Geometry: final body of the model. Coordinates: model frame, mm. Round coordinates to 2 decimals unless told otherwise and drop trailing zeros. Write each loop counter-clockwise with the first axis right and the second up, starting at its lowest first coordinate (ties: lowest second). Pieces come first, ordered by that corner, then holes. Notation, with made-up numbers: (-25.5, 72) - (26.5, 72) arc R20 ccw to (26.5, 93) - close; hole circle Ø2 at (42, 52.25). An arc over 180 degrees is marked (long way). Write each question's results on one line, items separated by ' | '.
from build123d import *

# Parameters (mm, degrees)
SKETCH_1_W          = 44.8
SKETCH_1_H          = 2000
EXTRUDE_1_DEPTH     = 10
CUT_EXTRUDE_2_DEPTH = 3329.04869605
EXTRUDE_2_DEPTH     = 44.8
CUT_EXTRUDE_3_DEPTH = 8.96


with BuildPart() as part:
    # 草图1 → 凸台-拉伸1 (new body)
    with BuildSketch(Plane(origin=(915.505475204, 0, 2515.33062051), x_dir=(-0.9396926207859093, 0, 0.3420201433256663), z_dir=(-0.3420201433256663, 0, -0.9396926207859093))):
        with Locations((-82.338659964, -943.731460395)):
            Rectangle(SKETCH_1_W, SKETCH_1_H)
    extrude(amount=-EXTRUDE_1_DEPTH)

    # 草图2 → 切除-拉伸2 (cut, through all)
    with BuildSketch(Plane(origin=(56.323916468, 0, -20.500229072), x_dir=(0.34202014332566644, 0, 0.9396926207859093), z_dir=(-0.9396926207859092, 0, 0.3420201433256664))):
        with BuildLine():
            Line((2678.733687242, 56.268539605), (2678.733687242, 49.653408924))
            Line((2678.733687242, 49.653408924), (2684.784186307, 49.653408924))
            ThreePointArc((2684.784186307, 49.653408924), (2684.783800485, 49.701723134), (2684.78264312, 49.750025021))
            Line((2684.78264312, 49.750025021), (2684.784186307, 56.268539605))
            Line((2684.784186307, 56.268539605), (2678.733687242, 56.268539605))
        make_face()
        with BuildLine():
            Line((2684.784186307, 49.653408924), (2678.733687242, 49.653408924))
            ThreePointArc((2678.733687242, 49.653408924), (2681.758936775, 46.628159392), (2684.784186307, 49.653408924))
        make_face()
    extrude(amount=-CUT_EXTRUDE_2_DEPTH, mode=Mode.SUBTRACT)

    # 草图3 → 凸台-拉伸2 (add)
    with BuildSketch(Plane(origin=(56.323916468, 0, -20.500229072), x_dir=(0.34202014332566644, 0, 0.9396926207859093), z_dir=(-0.9396926207859092, 0, 0.3420201433256664))):
        with BuildLine():
            Line((2678.733687242, 49.653408924), (2678.733687242, 56.268539605))
            Line((2678.733687242, 56.268539605), (2684.784186307, 56.268539605))
            Line((2684.784186307, 56.268539605), (2684.784186307, 49.653408924))
            ThreePointArc((2684.784186307, 49.653408924), (2681.758936775, 46.628159392), (2678.733687242, 49.653408924))
        make_face()
    extrude(amount=-EXTRUDE_2_DEPTH)

    # 草图4 → 切除-拉伸3 (cut)
    with BuildSketch(Plane(origin=(0, 56.268539605, 0), x_dir=(1, 0, 0), z_dir=(0, 1, 0))):
        Polygon((995.8288615, -2496.737076507), (996.29870781, -2496.566066436), (992.878506377, -2487.169140228), (992.408660067, -2487.340150299), align=None)
        Polygon((992.878506377, -2487.169140228), (996.29870781, -2496.566066436), (996.768554121, -2496.395056364), (993.348352687, -2486.998130156), align=None)
    extrude(amount=-CUT_EXTRUDE_3_DEPTH, mode=Mode.SUBTRACT)


solid = part.part
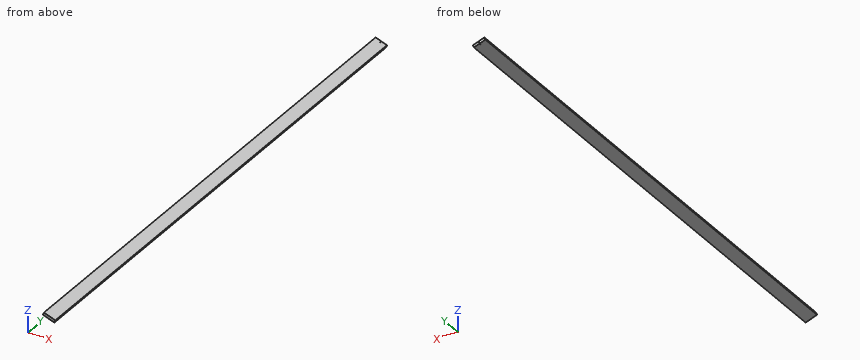
Q1. Section query A-A, the plane y = -304.5. Return loops of the section in (x, z), plus the area to 3 significant figures.
Answer block:
outline: (971.83, 2494.83) - (1013.93, 2479.51) - (1017.35, 2488.9) - (975.25, 2504.23) - close | area: 448 mm2
Q2. Pin query (flat end, axial travel): pin 1 (2 mm diameter, centred on x = 994.5, y = -587, fed in from -Z) (3 decimals); pin 2 (1.5 mm diameter, centred on x = 990, y = -1442.5, fed in from +Z); pin 3 (1.5 mm diameter, centred on x = 1004, y = -907.5, fed in from -Z). Return the tip coordinate at first contact, or that it passes through.
Answer block:
pin 1: z = 2486.215 | pin 2: z = 2499.13 | pin 3: z = 2482.85
Q3. Ray query, line 1 along Z through (x, y) = (990.5, -707.5); line 2 along Z through (x, y) = (997.5, -1129.5). Return the intervals inside material, ascending.
Answer block:
line 1: 2488.03 to 2498.68 | line 2: 2485.49 to 2496.13
